```python
from build123d import *

# Parameters (mm, degrees)
SKETCH1_W           = 58.8
SKETCH1_H           = 32
SKETCH1_R           = 1.55
BOSS_EXTRUDE1_DEPTH = 4.8
SKETCH2_R           = 3
CUT_EXTRUDE1_DEPTH  = 3
SKETCH3_W           = 58.8
SKETCH3_H           = 6
BOSS_EXTRUDE2_DEPTH = 16.8
CUT_EXTRUDE2_DEPTH  = 3
SKETCH5_R           = 1.6
CUT_EXTRUDE3_DEPTH  = 49.699075967


with BuildPart() as part:
    # Sketch1 → Boss-Extrude1 (new body)
    with BuildSketch(Plane(origin=(0, 0, 0), x_dir=(1, 0, 0), z_dir=(0, 1, 0))):
        Rectangle(SKETCH1_W, SKETCH1_H)
        with Locations(Location((-12.5, 12.5, 0), (0, 0, 270))):
            Circle(SKETCH1_R, mode=Mode.SUBTRACT)
        with Locations(Location((12.5, 12.5, 0), (0, 0, 270))):
            Circle(SKETCH1_R, mode=Mode.SUBTRACT)
        with Locations(Location((12.5, -12.5, 0), (0, 0, 270))):
            Circle(SKETCH1_R, mode=Mode.SUBTRACT)
        with Locations(Location((-12.5, -12.5, 0), (0, 0, 270))):
            Circle(SKETCH1_R, mode=Mode.SUBTRACT)
    extrude(amount=BOSS_EXTRUDE1_DEPTH)

    # Sketch2 → Cut-Extrude1 (cut)
    with BuildSketch(Plane.XZ):
        with Locations(Location((-12.5, 12.5, 0), (0, 0, 270))):
            Circle(SKETCH2_R)
        with Locations(Location((12.5, 12.5, 0), (0, 0, 270))):
            Circle(SKETCH2_R)
        with Locations(Location((12.5, -12.5, 0), (0, 0, 270))):
            Circle(SKETCH2_R)
        with Locations(Location((-12.5, -12.5, 0), (0, 0, 270))):
            Circle(SKETCH2_R)
    extrude(amount=-CUT_EXTRUDE1_DEPTH, mode=Mode.SUBTRACT)

    # Sketch3 → Boss-Extrude2 (add)
    with BuildSketch(Plane.XZ):
        with Locations((0, 19)):
            Rectangle(SKETCH3_W, SKETCH3_H)
    extrude(amount=-BOSS_EXTRUDE2_DEPTH)

    # Sketch4 → Cut-Extrude2 (cut)
    with BuildSketch(Plane(origin=(0, 0, 16), x_dir=(-1, 0, 0), z_dir=(0, 0, -1))):
        Polygon((-20.166838493, 10.8), (-21.783419246, 13.6), (-25.016580754, 13.6), (-26.633161507, 10.8), (-25.016580754, 8), (-21.783419246, 8), align=None)
    cut_extrude2 = extrude(amount=-CUT_EXTRUDE2_DEPTH, mode=Mode.SUBTRACT)

    # Sketch5 → Cut-Extrude3 (cut, through all)
    with BuildSketch(Plane(origin=(0, 0, 19), x_dir=(-1, 0, 0), z_dir=(0, 0, -1))):
        with Locations((-23.4, 10.8)):
            Circle(SKETCH5_R)
    cut_extrude3 = extrude(amount=-CUT_EXTRUDE3_DEPTH, mode=Mode.SUBTRACT)

    # Mirror1: Cut-Extrude2, Cut-Extrude3 across plane
    add(cut_extrude2.mirror(Plane(origin=(0, 0, 0), x_dir=(0, 0, 1), z_dir=(1, 0, 0))), mode=Mode.SUBTRACT)
    add(cut_extrude3.mirror(Plane(origin=(0, 0, 0), x_dir=(0, 0, 1), z_dir=(1, 0, 0))), mode=Mode.SUBTRACT)


solid = part.part
```
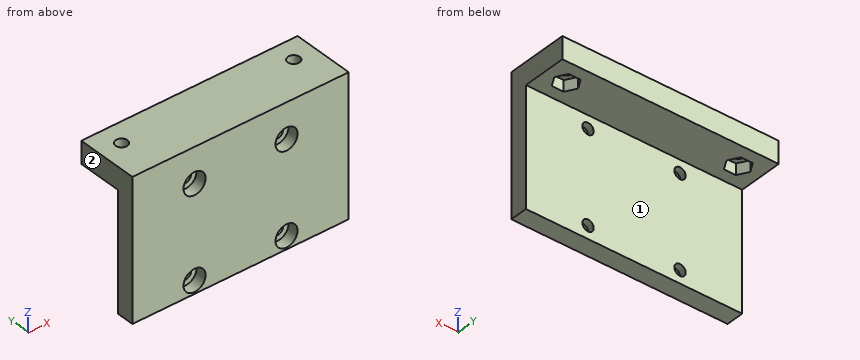
The listing builds one solid part. Answer for the finished solid, in the listing's coordinates (mm). Face numbers are marked on the shaded views. A direction names the side the tool comes from. Give positions to 0.01 mm unless a question says otherwise; leave off trailing zeros. Order: outer loops, then holes, each group sorted by start corner. A loop starts at its lowest first (then second) coordinate and runs counter-clockwise, first axis right, second up. Notation, with made-up numbers: (21, -7) - (75, -7) arc R14 cw to (75, 11) - close; hole circle Ø11 at (-15.5, 26). An arc over 180 degrees is marked (long way). Answer in a Markdown table with one row per item. Add a question column.
Q1. Which of the six approach directions +Z, -Z, +X, -X, +Y, -Y give full straight-line access (tool end or side, diameter ignored) to the marked faces 1 and 2?
Q2. The part is cut by section B-B (z = -12.5). Determine the outline of the cut face in (x, y).
Q3. Find the intervals of material crossed by line 1 along X through (y, z) = (3.7, -12.5); line 2 along Z through (x, y) = (-12.5, 4.1); line 3 along X through (y, z) = (2.3, -12.5), in increasing order. Write a range as [from, to].
Q4. The part is cut by section C-C (x = 23.4). Determine the outline of the cut face in (y, z), then the cut area to 3 significant figures.
Q5. The part is cut by section A-A (x = -12.5). Determine the outline of the cut face in (y, z).
Q6. The part is cut by section D-D (z = 1.5). Determine the outline of the cut face in (x, y).
Q7. Given P1, Ø1.7, axis at x = -22.5, y = 10, coming from the -Z side; P2, Ø3, axis at x = -12, z = 12.5, coming from the -Y side; P3, Ø6, axis at x = 22, y = 10, coming from the -Z side, each flat-ended and moving along its own axis, determine where each tip first touches the part or whether it passes through.
Determined:
| question | item | result |
|---|---|---|
| 1 | face 1 | -Z, +X, -X, +Y |
| 1 | face 2 | +Z, -Z, -X, +Y, -Y |
| 2 | outline | (-29.4, 0) - (-15.5, 0) - (-15.5, 3) - (-14.05, 3) - (-14.05, 4.8) - (-29.4, 4.8) - close; (-10.95, 3) - (-9.5, 3) - (-9.5, 0) - (9.5, 0) - (9.5, 3) - (10.95, 3) - (10.95, 4.8) - (-10.95, 4.8) - close; (14.05, 3) - (15.5, 3) - (15.5, 0) - (29.4, 0) - (29.4, 4.8) - (14.05, 4.8) - close |
| 3 | line 1 | x = [-29.4, -14.05], [-10.95, 10.95], [14.05, 29.4] |
| 3 | line 2 | z = [-16, -14.05], [-10.95, 10.95], [14.05, 22] |
| 3 | line 3 | x = [-29.4, -15.5], [-9.5, 9.5], [15.5, 29.4] |
| 4 | outline | (0, -16) - (4.8, -16) - (4.8, 16) - (8, 16) - (8, 19) - (9.2, 19) - (9.2, 22) - (0, 22) - close; (12.4, 19) - (13.6, 19) - (13.6, 16) - (16.8, 16) - (16.8, 22) - (12.4, 22) - close |
| 4 | area | 228 mm² |
| 5 | outline | (0, -16) - (4.8, -16) - (4.8, -14.05) - (3, -14.05) - (3, -15.5) - (0, -15.5) - close; (0, -9.5) - (3, -9.5) - (3, -10.95) - (4.8, -10.95) - (4.8, 10.95) - (3, 10.95) - (3, 9.5) - (0, 9.5) - close; (0, 15.5) - (3, 15.5) - (3, 14.05) - (4.8, 14.05) - (4.8, 16) - (16.8, 16) - (16.8, 22) - (0, 22) - close |
| 6 | outline | (-29.4, 0) - (29.4, 0) - (29.4, 4.8) - (-29.4, 4.8) - close |
| 7 | P1 | stops at z = 19 |
| 7 | P2 | stops at y = 3 |
| 7 | P3 | stops at z = 16 |
